Part print with two shaded views. Sizes in mm from the minimum x, y, z corner. Give positions to 0.01 mm unless a question says otherwise; leave off trailing zeros. Order: outer loops, then holes, each group sorted by start corner. A loop starts at its lowest first (then second) coordinate and runs counter-clockwise, first axis right, second up. Notation, with made-up numbers: (65, 89) -> (86, 89) arc R24 ccw to (86, 112) -> close; hole circle Ø10 at (-8, -25.75). An arc over 180 degrees is marked (long way). Write item = value, one per line. Start each with the question number.
Item 1: Band-saw the part on B-B on x = 120. Write the cut outline in (y, z).
Item 2: Drill centre lines: line 1 along X through (y, z) = (2.8, 8); line 2 along Z through (x, y) = (120, 4.05); line 3 along Z through (x, y) = (8.5, 3.3). Where is each one in solid material? Low to high.
Item 3: Band-saw the part on A-A on z = 8. Write the cut outline in (x, y), plus the area to 3 significant figures.
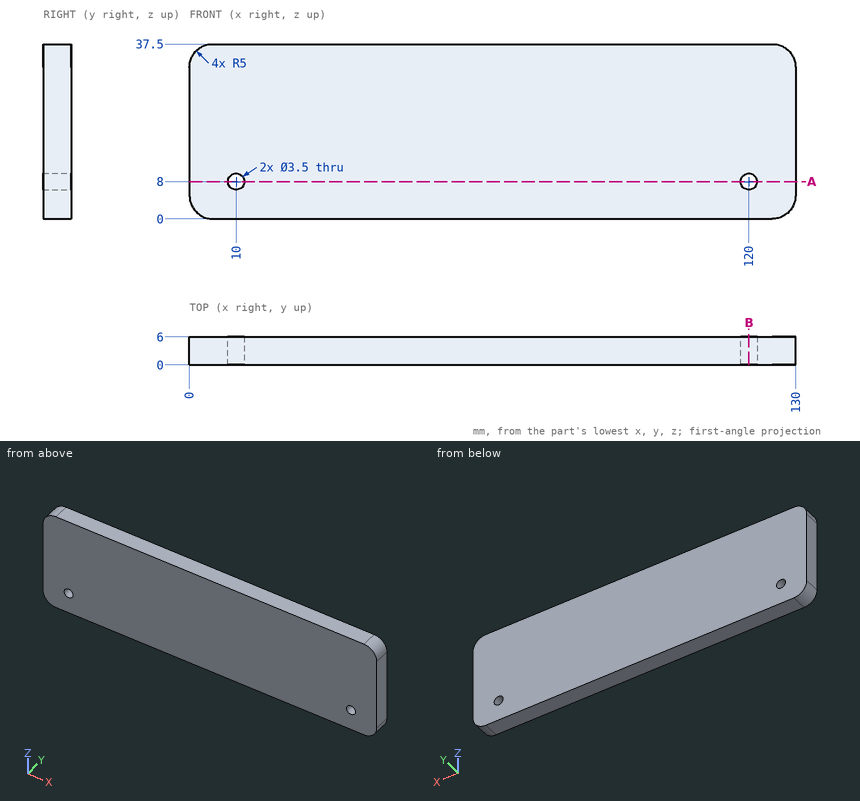
Values found:
q1.outline = (0, 0) -> (6, 0) -> (6, 6.25) -> (0, 6.25) -> close; (0, 9.75) -> (6, 9.75) -> (6, 37.5) -> (0, 37.5) -> close
q2.line_1 = 0 to 8.25, 11.75 to 118.25, 121.75 to 130
q2.line_2 = 0 to 6.25, 9.75 to 37.5
q2.line_3 = 0 to 7.1, 8.9 to 37.5
q3.outline = (0, 0) -> (8.25, 0) -> (8.25, 6) -> (0, 6) -> close; (11.75, 0) -> (118.25, 0) -> (118.25, 6) -> (11.75, 6) -> close; (121.75, 0) -> (130, 0) -> (130, 6) -> (121.75, 6) -> close
q3.area = 738 mm^2
